Build history of the part. All positions in model axes, mm. Face numbers are marked on the shaded views. A direction names the side the tool comes from. Round coordinates to 2 decimals unless told otherwise and drop trailing zeros. Loops run counter-clockwise (first coordinate to the right, second up) from the corner with the lowest first, then second, coordinate; pieces in that order, holes last.
from build123d import *

# Parameters (mm, degrees)
BOSS_EXTRUDE1_DEPTH = 75
SHELL1_T            = 10


with BuildPart() as part:
    # Sketch1 → Boss-Extrude1 (new body)
    with BuildSketch(Plane(origin=(0, 0, 0), x_dir=(1, 0, 0), z_dir=(0, 1, 0))):
        with BuildLine():
            Line((-317.803806735, 29.4427191), (-350.72176741, 0))
            Line((-350.72176741, 0), (-317.803806735, -29.4427191))
            ThreePointArc((-317.803806735, -29.4427191), (-280.622457508, -52.100683076), (-237.803806735, -60))
            Line((-237.803806735, -60), (-57.803806735, -60))
            ThreePointArc((-57.803806735, -60), (-43.661671111, -54.142135624), (-37.803806735, -40))
            Line((-37.803806735, -40), (-37.803806735, 40))
            ThreePointArc((-37.803806735, 40), (-43.661671111, 54.142135624), (-57.803806735, 60))
            Line((-57.803806735, 60), (-237.803806735, 60))
            ThreePointArc((-237.803806735, 60), (-280.622457508, 52.100683076), (-317.803806735, 29.4427191))
        make_face()
    extrude(amount=BOSS_EXTRUDE1_DEPTH)

    # Shell1
    shell1_openings = [part.faces().sort_by_distance(p)[0] for p in [
        (-177.328233539, 75, 0),
    ]]
    offset(amount=SHELL1_T, openings=shell1_openings, kind=Kind.INTERSECTION)


solid = part.part
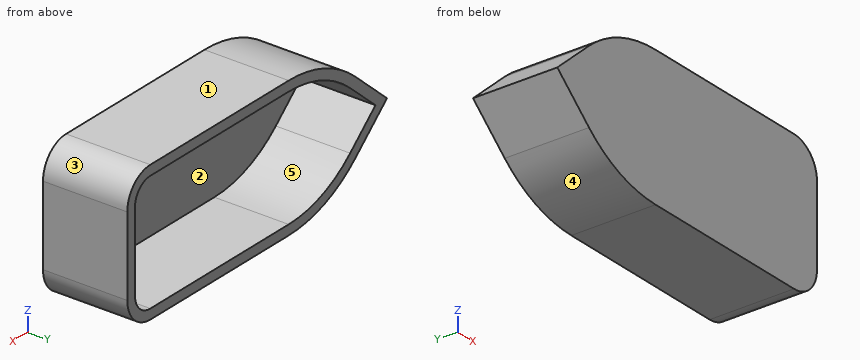
(1) Pull direction X, two halves, no side cores. Call the marked faces 3, 4 and 5: +X half, -X half, draft (parallel to the pull), parting line (faces both ways), or undercut.
Responses:
face 3: +X half
face 4: -X half
face 5: undercut
(2) Slice it at B-B on z = 24.5. List the corners of the cut face in (x, y).
Responses:
outline: (-338.33, -10) - (-27.8, -10) - (-27.8, 75) - (-37.8, 75) - (-37.8, 0) - (-323.33, 0) - (-323.33, 75) - (-338.33, 75) - close
(3) Pin check, flat tips, straight feed: P1, Ø8, axis at y = 13, z = 55, coming from the -X side; P2, Ø2, axis at x = -167.5, z = 19.5, coming from the +Y side; P3, Ø5, axis at y = 49.5, z = -29.5, coming from the -X side. Stop position of each tip, or through.
Responses:
P1: stops at x = -305.47
P2: stops at y = 0
P3: stops at x = -335.53
(4) Probe line 1 (Z direction, x = -119, y = 12); line 2 (Y direction, x = -77.5, z = 21); line 3 (Z direction, x = -342, y = 16). List the from-to ranges inside material, lowest first.
Responses:
line 1: z = -70 to -60, 60 to 70
line 2: y = -10 to 0
line 3: z = -21.22 to -7.8, 7.8 to 21.22
(5) Slice it at C-C on x = -340.5. List the corners of the cut face in (y, z), plus the area to 3 significant figures.
Responses:
outline: (-10, -22.56) - (75, -22.56) - (75, -9.14) - (0, -9.14) - (0, 9.14) - (75, 9.14) - (75, 22.56) - (-10, 22.56) - close
area: 2,460 mm2
(6) Slice it at A-A on y = 33. List the corners of the cut face in (x, z), plus the area to 3 significant figures.
Responses:
outline: (-365.72, 0) - (-324.47, -36.9) arc R130 ccw to (-237.8, -70) - (-57.8, -70) arc R30 ccw to (-27.8, -40) - (-27.8, 40) arc R30 ccw to (-57.8, 70) - (-237.8, 70) arc R130 ccw to (-324.47, 36.9) - close; hole (-350.72, 0) - (-317.8, -29.44) arc R120 ccw to (-237.8, -60) - (-57.8, -60) arc R20 ccw to (-37.8, -40) - (-37.8, 40) arc R20 ccw to (-57.8, 60) - (-237.8, 60) arc R120 ccw to (-317.8, 29.44) - close
area: 8,000 mm2
(7) Which spindle directions (+Z, -Z, +X, -X, +Y, -Y) get a long thin tool onto all of the face, cutting with end or side? Do the marked faces 1 and 2. Say none if no direction does.
Responses:
face 1: +Z, +X, -X, +Y, -Y
face 2: +Y
